from build123d import *

# Parameters (mm, degrees)
SKETCH_1_R      = 2
SKETCH_1_R_2    = 1.5
EXTRUDE_1_DEPTH = 12.5
SKETCH_2_R      = 2.25
EXTRUDE_2_DEPTH = 0.5
SKETCH_3_R      = 1.775
EXTRUDE_3_DEPTH = 1.25


with BuildPart() as part:
    # 스케치1 → 보스-돌출1 (new body, symmetric)
    with BuildSketch(Plane(origin=(0, 0, 0), x_dir=(1, 0, 0), z_dir=(0, 1, 0))):
        Circle(SKETCH_1_R)
        Circle(SKETCH_1_R_2, mode=Mode.SUBTRACT)
    extrude(amount=EXTRUDE_1_DEPTH, both=True)

    # 스케치2 → 보스-돌출2 (add)
    with BuildSketch(Plane(origin=(0, 12.5, 0), x_dir=(1, 0, 0), z_dir=(0, 1, 0))):
        Circle(SKETCH_2_R)
    extrude_2 = extrude(amount=EXTRUDE_2_DEPTH)

    # 스케치3 → 보스-돌출3 (add)
    with BuildSketch(Plane(origin=(0, 13, 0), x_dir=(1, 0, 0), z_dir=(0, 1, 0))):
        Circle(SKETCH_3_R)
    extrude_3 = extrude(amount=EXTRUDE_3_DEPTH)

    # 대칭 복사1: 보스-돌출2, 보스-돌출3 across plane
    add(extrude_2.mirror(Plane.ZX))
    add(extrude_3.mirror(Plane.ZX))


solid = part.part
CAD build for the part. Positions are in the model's coordinates, mm. A direction names the side the tool comes from. Give positions to 0.01 mm unless a question says otherwise; leave off trailing zeros. Write each loop counter-clockwise with the first axis right and the second up, starting at its lowest first coordinate (ties: lowest second). Pieces come first, ordered by that corner, then holes. Notation, with made-up numbers: M 77.25,-32 L 102.25,-32 A23 ccw 102.25,-2 Z; hole C -13.75,-19 d7. An arc over 180 degrees is marked long. Put each result on its own line as item: value. Start each with the question number.
(1) Flat gauge pins, fed straight in: pin 1 Ø1.5 at (y, z) = (-9.5, -0.5) entering from +X; pin 2 Ø1 at (x, y) = (0, -3.5) entering from +Z; pin 3 Ø2 at (x, y) = (0.5, -1.5) entering from -Z. Where does each tip first touch, or does it go through?
(2) Band-saw the part on B-B, the plane z = 0. Write the cut outline in (x, y) (3 decimals).
(3) Probe L1, parallel to Z at x = 0.1, y = -2.25; L2, parallel to Y at x = -1, z = -0.25. List the from-to ranges inside material, lowest first.
(4) Band-saw the part on A-A, the plane x = 0. Write the cut outline in (y, z) (3 decimals).
(5) Band-saw the part on C-C, the plane y = 4.5. Write the cut outline in (x, z), and give its area (3 significant figures).
(6) Which spindle directions (+Z, -Z, +X, -X, +Y, -Y) get a long thin tool onto all of the face, cutting with end or side? Do faces 4 (the face through (0, -13, -2)), 5 (the face through (-0.29, -12.75, -2.23)), 6 (the face through (0, -12.5, 0)), 7 (the face through (-0.23, 13.62, -1.76)), 8 (the face through (0, -14.25, 0)). Say none if no direction does.
(7) Mould opens along X. For faces 1 (the face through (0, 12.5, 0)), 2 (the face through (0, 14.25, 0)), 3 (the face through (0, 0, 2)) say: +X half, -X half, draft (parallel to the pull), parting line (faces both ways), or undercut.
Response values:
1. pin 1: stops at x = 2
1. pin 2: stops at z = 2
1. pin 3: stops at z = -2
2. outline: M -2.25,-13 L -1.775,-13 L -1.775,-14.25 L 1.775,-14.25 L 1.775,-13 L 2.25,-13 L 2.25,-12.5 L 2,-12.5 L 2,12.5 L 2.25,12.5 L 2.25,13 L 1.775,13 L 1.775,14.25 L -1.775,14.25 L -1.775,13 L -2.25,13 L -2.25,12.5 L -2,12.5 L -2,-12.5 L -2.25,-12.5 Z; hole M -1.5,-12.5 L 1.5,-12.5 L 1.5,12.5 L -1.5,12.5 Z
3. L1: z = -2 to -1.5, 1.5 to 2
3. L2: y = -14.25 to -12.5, 12.5 to 14.25
4. outline: M -14.25,-1.775 L -13,-1.775 L -13,-2.25 L -12.5,-2.25 L -12.5,-2 L 12.5,-2 L 12.5,-2.25 L 13,-2.25 L 13,-1.775 L 14.25,-1.775 L 14.25,1.775 L 13,1.775 L 13,2.25 L 12.5,2.25 L 12.5,2 L -12.5,2 L -12.5,2.25 L -13,2.25 L -13,1.775 L -14.25,1.775 Z; hole M -12.5,-1.5 L 12.5,-1.5 L 12.5,1.5 L -12.5,1.5 Z
5. outline: C 0,0 d4; hole C 0,0 d3
5. area: 5.50 mm2
6. face 4: -Y
6. face 5: +Y, -Y
6. face 6: none
6. face 7: +Y
6. face 8: +Z, -Z, +X, -X, -Y
7. face 1: undercut
7. face 2: draft
7. face 3: parting line
